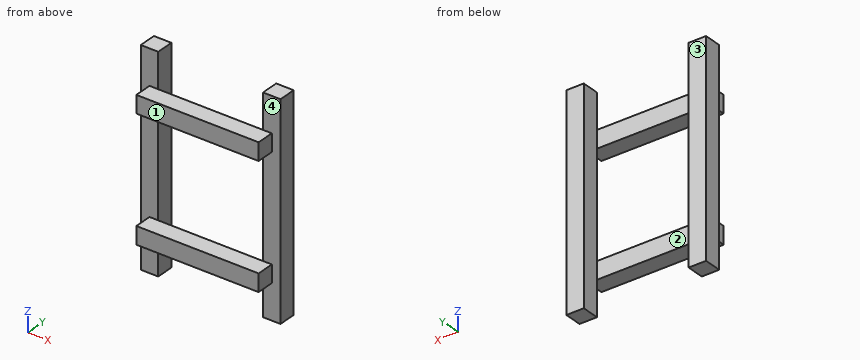
```python
from build123d import *

# Parameters (mm, degrees)
SKETCH1_W             = 50
SKETCH1_H             = 600
BOSS_EXTRUDE1_DEPTH   = 50
BOSS_EXTRUDE1_2_DEPTH = 50
SKETCH2_W             = 400
SKETCH2_H             = 50
BOSS_EXTRUDE2_DEPTH   = 50
SKETCH4_W             = 25
SKETCH4_H             = 400
CUT_EXTRUDE2_DEPTH    = 50


with BuildPart() as part:
    # Sketch1 → Boss-Extrude1 (new body)
    with BuildSketch(Plane(origin=(0, 0, 0), x_dir=(1, 0, 0), z_dir=(0, 1, 0))):
        with Locations((-106.932773109, -129.201680672)):
            Rectangle(SKETCH1_W, SKETCH1_H)
    extrude(amount=BOSS_EXTRUDE1_DEPTH)



with BuildPart() as body_2:
    # Sketch1 → Boss-Extrude1 2 (new body)
    with BuildSketch(Plane(origin=(0, 0, 0), x_dir=(1, 0, 0), z_dir=(0, 1, 0))):
        with Locations((243.067226891, -129.201680672)):
            Rectangle(SKETCH1_W, SKETCH1_H)
    extrude(amount=BOSS_EXTRUDE1_2_DEPTH)


with BuildPart() as part_1:
    add(part.part)

    add(body_2.part)  # Boss-Extrude2 merges body 2
    # Sketch2 → Boss-Extrude2 (add)
    with BuildSketch(Plane(origin=(0, 0, 0), x_dir=(-1, 0, 0), z_dir=(0, -1, 0))):
        with Locations((-68.067226891, -304.201680672)):
            Rectangle(SKETCH2_W, SKETCH2_H)
        with Locations((-68.067226891, 45.798319328)):
            Rectangle(SKETCH2_W, SKETCH2_H)
    extrude(amount=BOSS_EXTRUDE2_DEPTH)

    # Sketch4 → Cut-Extrude2 (cut)
    with BuildSketch(Plane(origin=(0, -50, 0), x_dir=(-1, 0, 0), z_dir=(0, -1, 0))):
        with Locations((-255.567226891, -129.201680672)):
            Rectangle(SKETCH4_W, SKETCH4_H)
        with Locations((119.432773109, -129.201680672)):
            Rectangle(SKETCH4_W, SKETCH4_H)
    extrude(amount=-CUT_EXTRUDE2_DEPTH, mode=Mode.SUBTRACT)


solid = part_1.part
```
The model under review builds one solid part; all positions refer to its coordinate system, in mm. Face numbers are marked on the shaded views. A direction names the side the tool comes from. Coordinates: 2 decimals unless noted, no trailing zeros. Write each loop counter-clockwise with the first axis right and the second up, starting at its lowest first coordinate (ties: lowest second). Pieces come first, ordered by that corner, then holes. Notation, with made-up numbers: (1.5, 5.25) - (35.5, 5.25) arc R4 ccw to (35.5, 11.25) - close; hole circle Ø9 at (72.5, 57.25). An arc over 180 degrees is marked (long way). Answer in a Markdown table with one row per item. Add a question column.
Q1. Consider section A-A on y = 13. Give the boundary of the cut face in (x, z), then the cut area to 3 significant figures.
Q2. Consider section B-B on z = 372. Give the boundary of the cut face in (x, y), then the cut area to 3 significant figures.
Q3. For the marked faces 1 and 2, list the 3-axis set-ups (+Z, -Z, +X, -X, +Y, -Y) from which the entire face can be reached by the end or side of a thin tool; tool diameter is ignored.
Q4. To check wall thickness, follow line 1 along X through (y, z) = (13.5, 118.5); line 2 along Z through (x, y) = (134.5, -40); line 3 along Y through (x, z) = (-108.5, 369). State the ranges of each line that lie inside material, in increasing order. Write a range as from..to.
Q5. Draft analysis for pull direction Z (two halves, no side actions). For the marked faces 3 and 4, state which applies: +Z half, -Z half, draft (parallel to the pull), parting line (faces both ways), or undercut.
Q6. Consider section C-C on x = 225. Give the boundary of the cut face in (y, z).
Q7. Clearance check with flat-ended pins moving along their axes: pin 1 (25 mm diameter, centred on y = -26.5, z = -57, fed in from +X); pin 2 (25 mm diameter, centred on x = 60, y = -29, fed in from +Z); pin 3 (15 mm diameter, centred on x = 64.5, z = 301, fed in from +Y). State where each tip first meets the part, or that it passes through.
Answers below:
| question | item | result |
|---|---|---|
| 1 | outline | (-131.93, -170.8) - (-81.93, -170.8) - (-81.93, 429.2) - (-131.93, 429.2) - close; (218.07, -170.8) - (268.07, -170.8) - (268.07, 429.2) - (218.07, 429.2) - close |
| 1 | area | 60,000 mm² |
| 2 | outline | (-131.93, 0) - (-81.93, 0) - (-81.93, 50) - (-131.93, 50) - close; (218.07, 0) - (268.07, 0) - (268.07, 50) - (218.07, 50) - close |
| 2 | area | 5,000 mm² |
| 3 | face 1 | +Z, -Z, +X, -X, -Y |
| 3 | face 2 | +Z, -Z, +Y |
| 4 | line 1 | -131.93..-81.93, 218.07..268.07 |
| 4 | line 2 | -70.8..-20.8, 279.2..329.2 |
| 4 | line 3 | 0..50 |
| 5 | face 3 | draft |
| 5 | face 4 | undercut |
| 6 | outline | (-50, -70.8) - (0, -70.8) - (0, -170.8) - (50, -170.8) - (50, 429.2) - (0, 429.2) - (0, 329.2) - (-50, 329.2) - (-50, 279.2) - (0, 279.2) - (0, -20.8) - (-50, -20.8) - close |
| 7 | pin 1 | x = 243.07 |
| 7 | pin 2 | z = 329.2 |
| 7 | pin 3 | y = 0 |
